Verification items for the finished model (mm, model axes). A direction names the side the tool comes from. Round coordinates to 2 decimals unless told otherwise and drop trailing zeros. Loops run counter-clockwise (first coordinate to the right, second up) from the corner with the lowest first, then second, coordinate; pieces in that order, holes last. Notation, with made-up numbers: (89.25, 65.25) -> (119.25, 65.25) arc R29 cw to (119.25, 94.25) -> close; hole circle Ø5 at (-39.5, 20.5). An arc over 180 degrees is marked (long way). Use CSV: the item, a comma, the result in double quotes. Start each with the question number.
```python
from build123d import *

# Parameters (mm, degrees)
SKETCH1_W           = 155.7
SKETCH1_H           = 155.7
BOSS_EXTRUDE2_DEPTH = 12
SKETCH2_W           = 18
SKETCH2_H           = 18
BOSS_EXTRUDE3_DEPTH = 38.1
SKETCH3_W           = 5.08
SKETCH3_H           = 3.048
BOSS_EXTRUDE4_DEPTH = 127
CHAMFER1_SIZE       = 0.508
CHAMFER1_SIZE2      = 0.03552282
CHAMFER2_SIZE       = 0.508
CHAMFER2_SIZE2      = 0.03552282
SKETCH4_W           = 5.334
SKETCH4_H           = 3.175
CUT_EXTRUDE3_DEPTH  = 149.86
SHELL1_START        = -20.543212121
SHELL1_DEPTH        = 152.144
SHELL1_2_OUTLINE_W  = 39.878
SHELL1_2_OUTLINE_H  = 14.444
SHELL1_2_DEPTH      = 14.444
SHELL1_START_2      = 129.316787879
SHELL1_3_OUTLINE_W  = 6.731
SHELL1_3_OUTLINE_H  = 5.334
SHELL1_3_DEPTH      = 2.284
FILLET1_R           = 1.27


# Read off the part's stored shape, not the designer's step: Shell1
with BuildPart() as part:
    # Sketch1 → Boss-Extrude2 (new body)
    with BuildSketch(Plane(origin=(0, 0, 0), x_dir=(1, 0, 0), z_dir=(0, 1, 0))):
        with Locations((55.528787879, -61.975)):
            Rectangle(SKETCH1_W, SKETCH1_H)
    extrude(amount=BOSS_EXTRUDE2_DEPTH)

    # Sketch2 → Boss-Extrude3 (add)
    with BuildSketch(Plane(origin=(0, 12, 0), x_dir=(1, 0, 0), z_dir=(0, 1, 0))):
        with Locations((-13.321212121, -130.825)):
            Rectangle(SKETCH2_W, SKETCH2_H)
    extrude(amount=BOSS_EXTRUDE3_DEPTH)

    # Sketch3 → Boss-Extrude4 (add)
    with BuildSketch(Plane.XY.offset(139.825)):
        with Locations((135.918787879, 6)):
            Rectangle(SKETCH3_W, SKETCH3_H)
    extrude(amount=-BOSS_EXTRUDE4_DEPTH)

    # Chamfer1
    chamfer1_edges = [part.edges().sort_by_distance(p)[0] for p in [
        (138.458787879, 7.524, 76.325),
    ]]
    chamfer1_side = [part.faces().sort_by_distance(p)[0] for p in [
        (135.918787879, 7.524, 76.325),
    ]]
    chamfer(chamfer1_edges, length=CHAMFER1_SIZE, length2=CHAMFER1_SIZE2, reference=chamfer1_side[0])

    # Chamfer2
    chamfer2_edges = [part.edges().sort_by_distance(p)[0] for p in [
        (138.458787879, 4.476, 76.325),
    ]]
    chamfer2_side = [part.faces().sort_by_distance(p)[0] for p in [
        (135.918787879, 4.476, 76.325),
    ]]
    chamfer(chamfer2_edges, length=CHAMFER2_SIZE, length2=CHAMFER2_SIZE2, reference=chamfer2_side[0])

    # Sketch4 → Cut-Extrude3 (cut)
    with BuildSketch(Plane.ZY.offset(22.321212121)):
        with Locations((-13.208, 6)):
            Rectangle(SKETCH4_W, SKETCH4_H)
    extrude(amount=-CUT_EXTRUDE3_DEPTH, mode=Mode.SUBTRACT)

    # Shell1 outline → Shell1 (cut)
    with BuildSketch(Plane.YZ.offset(SHELL1_START)):
        Polygon((10.222, 138.047), (1.778, 138.047), (1.778, -14.097), (2.6345, -14.097), (2.6345, -8.763), (9.3655, -8.763), (9.3655, -14.097), (10.222, -14.097), align=None)
    extrude(amount=SHELL1_DEPTH, mode=Mode.SUBTRACT)

    # Shell1 2 outline → Shell1 2 (cut)
    with BuildSketch(Plane.YZ.offset(SHELL1_START)):
        with Locations((30.161, 130.825)):
            Rectangle(SHELL1_2_OUTLINE_W, SHELL1_2_OUTLINE_H)
    extrude(amount=SHELL1_2_DEPTH, mode=Mode.SUBTRACT)

    # Shell1 3 outline → Shell1 3 (cut)
    with BuildSketch(Plane.YZ.offset(SHELL1_START_2)):
        with Locations((6, -11.43)):
            Rectangle(SHELL1_3_OUTLINE_W, SHELL1_3_OUTLINE_H)
    extrude(amount=SHELL1_3_DEPTH, mode=Mode.SUBTRACT)

    # Fillet1
    fillet1_edges = [part.edges().sort_by_distance(p)[0] for p in [
        (-22.321212121, 50.1, 130.825),
        (-13.321212121, 50.1, 139.825),
        (-4.321212121, 50.1, 130.825),
        (-13.321212121, 50.1, 121.825),
    ]]
    fillet(fillet1_edges, radius=FILLET1_R)


solid = part.part
```
Q1. Cross-section at B-B (y = 19). Record the boundary of the cut face in (x, z) (3 decimals), and give its area (3 significant figures).
Q2. Thickness scan on L1, parallel to Y at x = 67, z = 35.5; L2, parallel to X at y = 10.5, z = 126.5; L3, parallel to Z at x = 77, y = 8 (3 decimals). Record the ranges inside material, lowest first. Write a range as from..to.
Q3. Depth check by flat-ended pin: pin 1 Ø6 at (x, z) = (25, 102.5) entering from +Y; pin 2 Ø1.5 at (y, z) = (25, 123) entering from +X; pin 3 Ø1.6 at (y, z) = (6.5, -12.5) entering from +X. Enter the tip coordinate at first touch or a pass-through.
Q4. Tool access check on faces 4 (the face through (55, 10, -14.097)), 5 (the face through (-4.321, 30, 131)), 6 (the face through (-13, 30, 123.603)), 7 (the face through (-13, 30, 121.825)). Record the directions out of +Z, -Z, +X, -X, +Y, -Y that give a thin tool (end or side, any length) a straight path to the whole face; none if there is none.
Q5. Release check for a two-part mould opening along Y. For faces 1 (the face through (131.601, 6, 63)), 2 (the face through (54, 3, -15.875)), 3 (the face through (54, 0, 61)) record: +Y half, -Y half, draft (parallel to the pull), parting line (faces both ways), or undercut.
Q6. Cross-section at C-C (x = 96.5). Record the boundary of the cut face in (y, z) (1 decimal), and give its area (3 significant figures).
Q7. Cross-section at A-A (z = 90). Record the boundary of the cut face in (x, y).
Answer list:
1,outline,"(-22.321, 121.825) -> (-4.321, 121.825) -> (-4.321, 139.825) -> (-22.321, 139.825) -> close; hole (-20.543, 123.603) -> (-6.099, 123.603) -> (-6.099, 138.047) -> (-20.543, 138.047) -> close"
1,area,"115 mm2"
2,L1,"y = 0..1.78, 10.22..12"
2,L2,"x = -22.32..-20.54, -6.1..133.38"
2,L3,"z = -15.875..-8.763, 138.047..139.825"
3,pin 1,"stops at y = 12"
3,pin 2,"stops at x = -4.32"
3,pin 3,"stops at x = 133.38"
4,face 4,"none"
4,face 5,"+Z, -Z, +X, +Y"
4,face 6,"+Y"
4,face 7,"-Z, +X, -X, +Y"
5,face 1,"undercut"
5,face 2,"draft"
5,face 3,"-Y half"
6,outline,"(0, -15.9) -> (4.4, -15.9) -> (4.4, -10.5) -> (7.6, -10.5) -> (7.6, -15.9) -> (12, -15.9) -> (12, 139.8) -> (0, 139.8) -> close; hole (1.8, -14.1) -> (2.6, -14.1) -> (2.6, -8.8) -> (9.4, -8.8) -> (9.4, -14.1) -> (10.2, -14.1) -> (10.2, 138) -> (1.8, 138) -> close"
6,area,"603 mm2"
7,outline,"(-22.32, 0) -> (133.38, 0) -> (133.38, 4.48) -> (137.95, 4.48) -> (138.46, 4.51) -> (138.46, 7.49) -> (137.95, 7.52) -> (133.38, 7.52) -> (133.38, 12) -> (-22.32, 12) -> close; hole (-20.54, 1.78) -> (131.6, 1.78) -> (131.6, 10.22) -> (-20.54, 10.22) -> close"
